Part print with two shaded views. Sizes in mm from the minimum x, y, z corner. Round coordinates to 2 decimals unless told otherwise and drop trailing zeros. Loops run counter-clockwise (first coordinate to the right, second up) from the corner with the lowest first, then second, coordinate; pieces in that order, holes last. Notation, with made-up numbers: (-28.5, 38.5) - (-4.5, 38.5) arc R25 ccw to (-4.5, 51.5) - close; hole circle Ø11 at (67.5, 44.25). An arc over 180 degrees is marked (long way). Use a Markdown table: item, result.
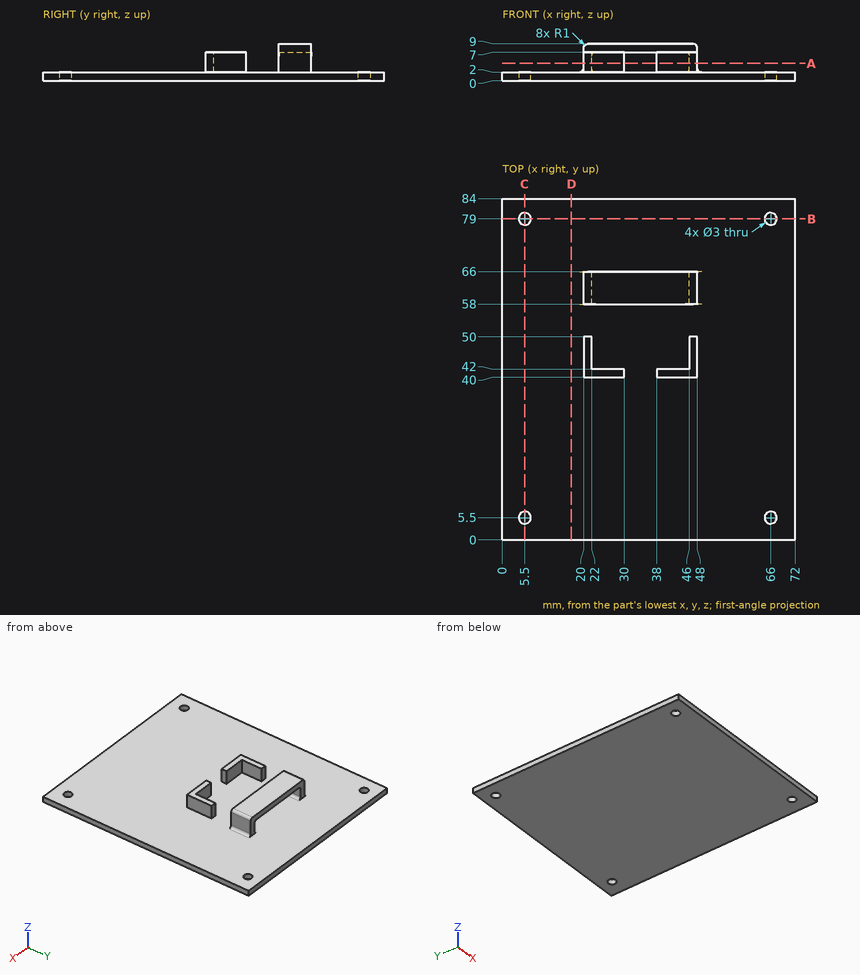
Q1. Drop flat-ended pins along their axis: pin 1 (1 mm diameter, centred on x = 10, y = 63, fed in from +Z); pin 2 (8 mm diameter, centred on x = 45, y = 46.5, fed in from +Z); pin 3 (2 mm diameter, centred on y = 41.5, z = 5, fed in from +X). Give the stop position or say it passes through.
Results found:
| item | result |
|---|---|
| pin 1 | stops at z = 2 |
| pin 2 | stops at z = 7 |
| pin 3 | stops at x = 48 |
Q2. Cut at C-C, the plane x = 5.5. List the corners of the cut face in (y, z).
Results found:
| item | result |
|---|---|
| outline | (0, 0) - (4, 0) - (4, 2) - (0, 2) - close; (7, 0) - (77.5, 0) - (77.5, 2) - (7, 2) - close; (80.5, 0) - (84, 0) - (84, 2) - (80.5, 2) - close |
Q3. Cut at B-B, the plane y = 79. List the corners of the cut face in (x, z).
Results found:
| item | result |
|---|---|
| outline | (0, 0) - (4, 0) - (4, 2) - (0, 2) - close; (7, 0) - (64.5, 0) - (64.5, 2) - (7, 2) - close; (67.5, 0) - (72, 0) - (72, 2) - (67.5, 2) - close |
Q4. Cut at D-D, the plane x = 17. List the corners of the cut face in (y, z), plus the area to 3 significant figures.
Results found:
| item | result |
|---|---|
| outline | (0, 0) - (84, 0) - (84, 2) - (0, 2) - close |
| area | 168 mm2 |
Q5. Probe line 1 (Y direction, x = 66, z = 1.1); line 2 (X direction, y = 79, z = 0.4); line 3 (X direction, y = 43.5, z = 4.25). List the from-to ranges inside material, lowest first.
Results found:
| item | result |
|---|---|
| line 1 | y = 0 to 4, 7 to 77.5, 80.5 to 84 |
| line 2 | x = 0 to 4, 7 to 64.5, 67.5 to 72 |
| line 3 | x = 20 to 22, 46 to 48 |
Q6. Cut at A-A, the plane z = 4.25. List the corners of the cut face in (x, y), plus the area to 3 significant figures.
Results found:
| item | result |
|---|---|
| outline | (20, 40) - (30, 40) - (30, 42) - (22, 42) - (22, 50) - (20, 50) - close; (20, 58) - (22, 58) - (22, 66) - (20, 66) - close; (38, 40) - (48, 40) - (48, 50) - (46, 50) - (46, 42) - (38, 42) - close; (46, 58) - (48, 58) - (48, 66) - (46, 66) - close |
| area | 104 mm2 |
